Read the model definition and answer for the solid it produces. Units are mm, in the model's axes. Coordinates: 2 decimals unless noted, no trailing zeros. Loops run counter-clockwise (first coordinate to the right, second up) from the corner with the lowest first, then second, coordinate; pieces in that order, holes last.
Q1. Straight lines are drawn through the part: line 1 (Z direction, x = -16, y = 1.4); line 2 (X direction, y = 1.7, z = -29.5); line 3 (X direction, y = 1.15, z = -29). For each, find the intervals that lie inside material, in ascending order.
Q2. Section A-A (x = -16.5) is taken. Give the vertices of the cut face in (y, z).
Q3. Flat-ended cylindrical pins translate along their axes: P1, Ø0.9, axis at y = 1.5, z = -32, coming from the -X side; P2, Ø1.5, axis at x = -2, y = 1.5, coming from the -Z side; P3, Ø1.2, axis at x = -25, y = 1, coming from the +Z side. Find the tip coordinate at first contact, or state that the pin passes through.
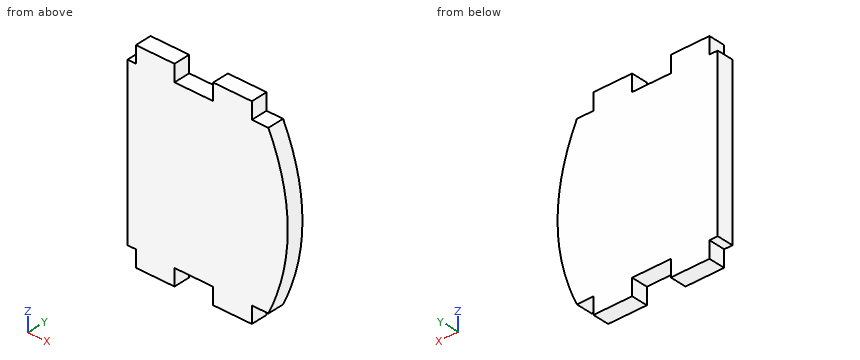
Autodesk Inventor part; units mm, degrees
ref_plane "YZ Plane" through (0, 0, 0) normal (1, 0, 0) x (0, 1, 0)
ref_plane "XZ Plane" through (0, 0, 0) normal (0, 1, 0) x (-1, 0, 0)
ref_plane "XY Plane" through (0, 0, 0) normal (0, 0, 1) x (1, 0, 0)
sketch "Esquisse1" plane through (0, 0, 0) normal (0, 1, 0) x (-1, 0, 0)
  line L0 (0, 0) -> (25.5, 0)
  line L1 (25.5, 0) -> (25.5, -30)
  line L2 (25.5, -30) -> (0, -30)
  line L3 (0, -30) -> (0, 0)
  line L4 (3, 0) -> (10, 0)
  line L5 (10, 0) -> (10, 3)
  line L6 (10, 3) -> (3, 3)
  line L7 (3, 3) -> (3, 0)
  line L8 (25.5, -15) -> (0, -15) construction
  line L9 (14, 0) -> (39.5, 0)
  line L10 (17, 0) -> (24, 0)
  line L11 (24, 0) -> (24, 3)
  line L12 (24, 3) -> (17, 3)
  line L13 (17, 3) -> (17, 0)
  line L14 (3, -30) -> (10, -30)
  line L15 (10, -30) -> (10, -33)
  line L16 (10, -33) -> (3, -33)
  line L17 (3, -33) -> (3, -30)
  line L18 (17, -30) -> (24, -30)
  line L19 (24, -30) -> (24, -33)
  line L20 (24, -33) -> (17, -33)
  line L21 (17, -33) -> (17, -30)
  line L22 (0, 0) -> (-7, -15) construction
  line L23 (-7, -15) -> (0, -30) construction
  spline S0 degree 2 poles (0, 0) (-7, -15) (0, -30) knots 1 1 1 2 2 2
  line L24 (-7, -15) -> (0, -15) construction
  point P0 (14, -30)
  dimension "d0" = 30
  dimension "d1" = 3
  dimension "d2" = 7
  dimension "d3" = 3
  dimension "d6" = 14
  dimension "d11" = 1.5
  dimension "d12" = 7
extrude "Plaque1" add sketch "Esquisse1" along normal blind 3
equation "\"d6\" = 2 * d2"
equation "\"LargeurGrugeage\" = Epaisseur"
equation "\"ProfondeurGrugeage\" = 0.5 * Epaisseur"
equation "\"TailleGrugeage\" = 4 * Epaisseur"
equation "\"RestesMinimum\" = 2 * Epaisseur"
equation "\"Rayondetransition\" = RayonPli"
equation "\"TailleRayonJacobi\" = RayonPli"
equation "\"TailleJeu\" = Epaisseur"
equation "\"d13\" = RayonPli"
properties part number "tip" material "Plastique PMMA"
Numbers:
1. line 1: z = -30 to 0
1. line 2: x = -25.5 to 0.23
1. line 3: x = -25.5 to 0.45
2. outline: (0, -30) - (3, -30) - (3, 0) - (0, 0) - close
3. P1: stops at x = -24
3. P2: stops at z = -30
3. P3: stops at z = 0
